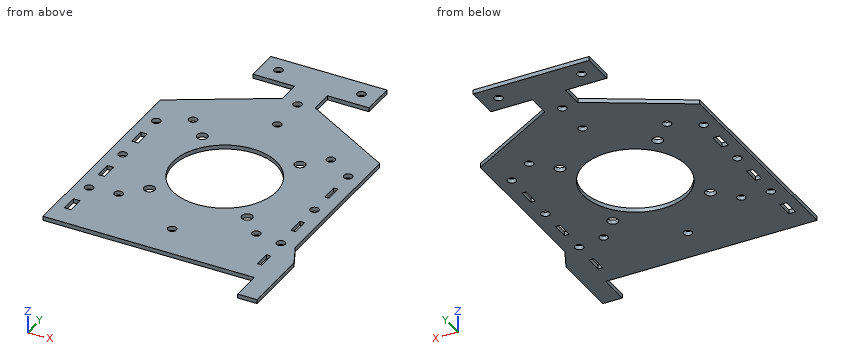
```python
from build123d import *

# Parameters (mm, degrees)
SKETCH_1_W      = 3.1
SKETCH_1_H      = 8.1
SKETCH_1_R      = 2.05
SKETCH_1_R_2    = 2.55
SKETCH_1_R_3    = 25
SKETCH_1_W_2    = 2.1
EXTRUDE_1_DEPTH = 2


with BuildPart() as part:
    # 草图1 → 凸台-拉伸1 (new body)
    with BuildSketch(Plane.XY):
        Polygon((52.9, -21.5), (52.9, 53.883164809), (8, 79.569735886), (8, 90.5), (28, 90.5), (28, 106.5), (-28, 106.5), (-28, 90.5), (-8, 90.5), (-8, 79.569735886), (-52.9, 53.883164809), (-52.9, -50.79), (-43.709229173, -50.79), (-34.403358285, -50.79), (48.918692166, -50.79), (48.918692166, -65.64215863), (58.26995581, -65.64215863), (58.26995581, -32.590877477), align=None)
        with Locations((-46.5, -36.5)):
            Rectangle(SKETCH_1_W, SKETCH_1_H, mode=Mode.SUBTRACT)
        with Locations((0, -33.5)):
            Circle(SKETCH_1_R, mode=Mode.SUBTRACT)
        with Locations((-46.5, -21.5)):
            Circle(SKETCH_1_R, mode=Mode.SUBTRACT)
        with Locations((-46.5, -6.5)):
            Rectangle(SKETCH_1_W, SKETCH_1_H, mode=Mode.SUBTRACT)
        with Locations((-33.234018716, -19.734018716)):
            Circle(SKETCH_1_R, mode=Mode.SUBTRACT)
        with Locations((-46.5, 8.5)):
            Circle(SKETCH_1_R, mode=Mode.SUBTRACT)
        with Locations((-23.57, -10.07)):
            Circle(SKETCH_1_R_2, mode=Mode.SUBTRACT)
        with Locations((0, 13.5)):
            Circle(SKETCH_1_R_3, mode=Mode.SUBTRACT)
        with Locations((46, -36.5)):
            Rectangle(SKETCH_1_W_2, SKETCH_1_H, mode=Mode.SUBTRACT)
        with Locations((23.57, -10.07)):
            Circle(SKETCH_1_R_2, mode=Mode.SUBTRACT)
        with Locations((33.234018716, -19.734018716)):
            Circle(SKETCH_1_R, mode=Mode.SUBTRACT)
        with Locations((46, -21.5)):
            Circle(SKETCH_1_R, mode=Mode.SUBTRACT)
        with Locations((46, -6.5)):
            Rectangle(SKETCH_1_W_2, SKETCH_1_H, mode=Mode.SUBTRACT)
        with Locations((46, 8.5)):
            Circle(SKETCH_1_R, mode=Mode.SUBTRACT)
        with Locations((-46.5, 23.5)):
            Rectangle(SKETCH_1_W, SKETCH_1_H, mode=Mode.SUBTRACT)
        with Locations((-46.5, 38.5)):
            Circle(SKETCH_1_R, mode=Mode.SUBTRACT)
        with Locations((-33.234018716, 46.734018716)):
            Circle(SKETCH_1_R, mode=Mode.SUBTRACT)
        with Locations((-23.57, 37.07)):
            Circle(SKETCH_1_R_2, mode=Mode.SUBTRACT)
        with Locations((0, 60.5)):
            Circle(SKETCH_1_R, mode=Mode.SUBTRACT)
        with Locations((0, 78.5)):
            Circle(SKETCH_1_R, mode=Mode.SUBTRACT)
        with Locations((-20, 98.5)):
            Circle(SKETCH_1_R, mode=Mode.SUBTRACT)
        with Locations((23.57, 37.07)):
            Circle(SKETCH_1_R_2, mode=Mode.SUBTRACT)
        with Locations((46, 23.5)):
            Rectangle(SKETCH_1_W_2, SKETCH_1_H, mode=Mode.SUBTRACT)
        with Locations((46, 38.5)):
            Circle(SKETCH_1_R, mode=Mode.SUBTRACT)
        with Locations((33.234018716, 46.734018716)):
            Circle(SKETCH_1_R, mode=Mode.SUBTRACT)
        with Locations((20, 98.5)):
            Circle(SKETCH_1_R, mode=Mode.SUBTRACT)
    extrude(amount=EXTRUDE_1_DEPTH)


solid = part.part
```
Can you work these out from the model? Positions are in its coordinate system, mm. Coordinates: 2 decimals unless noted, no trailing zeros. Loops run counter-clockwise (first coordinate to the right, second up) from the corner with the lowest first, then second, coordinate; pieces in that order, holes last.
Item 1: Please list where these lines run through material, in increasing order: L1, parallel to Y at x = 0, z = 1.55; L2, parallel to Y at x = 9, z = 1.6; L3, parallel to Y at x = -20.5, z = 1.9.
Answers below:
L1: y = -50.79 to -35.55, -31.45 to -11.5, 38.5 to 58.45, 62.55 to 76.45, 80.55 to 106.5
L2: y = -50.79 to -9.82, 36.82 to 79, 90.5 to 106.5
L3: y = -50.79 to -0.81, 27.81 to 72.42, 90.5 to 96.51, 100.49 to 106.5
Item 2: Suppose I cut it at B-B (x = 14). Please give me the cut outline in (y, z).
Answers below:
outline: (-50.79, 0) - (-7.21, 0) - (-7.21, 2) - (-50.79, 2) - close; (34.21, 0) - (76.14, 0) - (76.14, 2) - (34.21, 2) - close; (90.5, 0) - (106.5, 0) - (106.5, 2) - (90.5, 2) - close
Item 3: Suppose I cut it at D-D (z = 1). State how many separate pieces and enclosed holes the cut face has, then the cut area to 3 significant figures.
Answers below:
separate pieces: 1
enclosed holes: 26
area: 11,600 mm2
Item 4: Suppose I cut it at A-A (y = 13.5). Please give me the cut outline in (x, z), then the cut area to 3 significant figures.
Answers below:
outline: (-52.9, 0) - (-25, 0) - (-25, 2) - (-52.9, 2) - close; (25, 0) - (52.9, 0) - (52.9, 2) - (25, 2) - close
area: 112 mm2
Item 5: I'm going to push flat-ended pins straight in: pin 1 (1 mm diameter, centred on x = 46, z = 1.5, fed in from +Y); pin 2 (1 mm diameter, centred on x = -47, z = 1, fed in from +Y); pin 3 (2.5 mm diameter, centred on x = -46.5, y = 38.5, fed in from -Z); pin 4 (1 mm diameter, centred on x = 15.5, z = 1.5, fed in from -Y). Where does each tip first touch, or does it pass through?
Answers below:
pin 1: stops at y = 58.12
pin 2: stops at y = 57.54
pin 3: passes through
pin 4: stops at y = -50.79
Item 6: Suppose I cut it at C-C (x = -5). Please give me the cut outline in (y, z), then the cut area to 3 significant figures.
Answers below:
outline: (-50.79, 0) - (-10.99, 0) - (-10.99, 2) - (-50.79, 2) - close; (37.99, 0) - (106.5, 0) - (106.5, 2) - (37.99, 2) - close
area: 217 mm2
